Design review of the part built by this model. Coordinates are the model's own, in mm. A direction names the side the tool comes from. Coordinates: 2 decimals unless noted, no trailing zeros. Order: outer loops, then holes, each group sorted by start corner. A loop starts at its lowest first (then second) coordinate and runs counter-clockwise, first axis right, second up. Notation, with made-up numbers: M 31,-4.5 L 82,-4.5 A35 ccw 82,33.5 Z; hole C 25,16 d3. An arc over 180 degrees is marked long. Answer as a JSON object with one key per item and string values.
Autodesk Inventor part; units mm, degrees
ref_plane "Midplane" through (-32.0857, 98.175, 0) normal (0, -1, 0) x (1, 0, 0)
ref_plane "Work Plane3" through (-26.5857, 212.35, 16) normal (1, 0, 0) x (0, 0, -1)
ref_plane "YZ Plane" through (0, 0, 0) normal (1, 0, 0) x (0, 1, 0)
sketch "Sketch2" plane through (0, 0, 0) normal (0, 0, 1) x (1, 0, 0)
  line L0 (-32.0857, 0) -> (0, 0)
  line L1 (0, 0) -> (0, 19.635)
  line L2 (0, 19.635) -> (-32.0857, 19.635)
  spline S0 degree 3 poles (-32.0857, 19.635) (-32.0786, 19.6019) (-32.0585, 19.4984) (-32.0378, 19.3226) (-32.0222, 19.1083) (-32.0293, 18.8935) (-32.0484, 18.6795) (-32.102, 18.3981) (-32.1765, 18.0482) (-32.2416, 17.6965) (-32.2997, 17.416) (-32.364, 17.211) (-32.4396, 17.0099) (-32.536, 16.8179) (-32.6409, 16.6304) (-32.7641, 16.4543) (-32.8983, 16.2866) (-33.043, 16.1278) (-33.201, 15.9822) (-33.3669, 15.8459) (-33.5414, 15.7205) (-33.7857, 15.5713) (-34.1055, 15.4094) (-34.509, 15.2608) (-34.9249, 15.1525) (-35.3479, 15.078) (-35.7753, 15.0341) (-36.2047, 15.0215) (-36.6341, 15.0313) (-37.0623, 15.0646) (-37.3462, 15.1014) (-37.4881, 15.1198) knots -0.847201 -0.847201 -0.847201 -0.847201 -0.83705 -0.815587 -0.794126 -0.772659 -0.751201 -0.729734 -0.686802 -0.64387 -0.622403 -0.600945 -0.579478 -0.558017 -0.536554 -0.515088 -0.49363 -0.472163 -0.450698 -0.429238 -0.407769 -0.386302 -0.343394 -0.300476 -0.257562 -0.214646 -0.17172 -0.12879 -0.085861 -0.04293 0 0 0 0
  spline S1 degree 3 poles (-37.4881, 15.1198) (-37.594, 15.1249) (-37.8057, 15.1352) (-38.2295, 15.119) (-38.7575, 15.0717) (-39.3865, 14.9771) (-40.0103, 14.8535) (-40.6285, 14.7043) (-41.2408, 14.5326) (-41.847, 14.3405) (-42.4469, 14.1297) (-43.0405, 13.9015) (-43.6276, 13.6572) (-44.2081, 13.3977) (-44.782, 13.1239) (-45.3493, 12.8367) (-45.9097, 12.5363) (-46.4639, 12.2246) (-46.8275, 12.0066) (-47.0092, 11.8976) knots -1.017256 -1.017256 -1.017256 -1.017256 -0.985476 -0.953687 -0.890117 -0.826542 -0.762964 -0.699386 -0.635807 -0.572227 -0.508647 -0.445066 -0.381486 -0.317905 -0.254324 -0.190743 -0.127162 -0.063581 0 0 0 0
  arc A0 (-47.0092, 11.8976) -> (-47.0092, 7.7374) centre (9.2023, 9.8175) ccw
  spline S2 degree 3 poles (-47.0092, 7.7374) (-46.8275, 7.6284) (-46.4639, 7.4104) (-45.9097, 7.0987) (-45.3493, 6.7983) (-44.782, 6.5111) (-44.2081, 6.2373) (-43.6276, 5.9778) (-43.0405, 5.7335) (-42.4469, 5.5053) (-41.847, 5.2945) (-41.2408, 5.1024) (-40.6285, 4.9307) (-40.0103, 4.7815) (-39.3865, 4.6579) (-38.7575, 4.5633) (-38.2295, 4.516) (-37.8057, 4.4998) (-37.594, 4.5101) (-37.4881, 4.5152) knots -1.017256 -1.017256 -1.017256 -1.017256 -0.953675 -0.890094 -0.826513 -0.762932 -0.699351 -0.63577 -0.572189 -0.508609 -0.445029 -0.381449 -0.31787 -0.254291 -0.190714 -0.127139 -0.063568 -0.03178 0 0 0 0
  spline S3 degree 3 poles (-37.4881, 4.5152) (-37.3462, 4.5336) (-37.0623, 4.5704) (-36.6341, 4.6037) (-36.2047, 4.6135) (-35.7753, 4.6009) (-35.3479, 4.557) (-34.9249, 4.4825) (-34.509, 4.3742) (-34.1055, 4.2256) (-33.7857, 4.0637) (-33.5414, 3.9145) (-33.3669, 3.7891) (-33.201, 3.6528) (-33.043, 3.5072) (-32.8983, 3.3484) (-32.7641, 3.1807) (-32.6409, 3.0046) (-32.536, 2.8171) (-32.4396, 2.6251) (-32.364, 2.424) (-32.2997, 2.219) (-32.2416, 1.9385) (-32.1765, 1.5868) (-32.102, 1.2369) (-32.0484, 0.9555) (-32.0293, 0.7415) (-32.0222, 0.5267) (-32.0378, 0.3124) (-32.0585, 0.1366) (-32.0786, 0.0331) (-32.0857, 0) knots -1.373604 -1.373604 -1.373604 -1.373604 -1.330674 -1.287743 -1.244814 -1.201884 -1.158958 -1.116042 -1.073128 -1.03021 -0.987302 -0.965835 -0.944366 -0.922906 -0.901441 -0.879974 -0.858516 -0.83705 -0.815587 -0.794126 -0.772659 -0.751201 -0.729734 -0.686802 -0.64387 -0.622403 -0.600945 -0.579478 -0.558017 -0.536554 -0.526403 -0.526403 -0.526403 -0.526403
extrude "Extrusion1" add sketch "Sketch2" along normal blind 16
pattern_linear "Rectangular Pattern1" count 10 spacing 19.635 along (0, 1, 0) of "Extrusion1"
sketch "Sketch5" plane through (-32.0857, 0, 0) normal (0, -1, 0) x (1, 0, 0)
  line L0 (32.0857, 0) -> (32.0857, 16)
  line L1 (0, 16) -> (32.0857, 16)
  line L2 (0, 0) -> (32.0857, 0)
  line L3 (0, 0) -> (0, 16)
  line L4 (0, 16) -> (8, 16)
  line L5 (8, 16) -> (8, 0) construction
  line L6 (8, 0) -> (0, 0)
  line L7 (0, 0) -> (0, 16)
  line L8 (8, 16) -> (10.5, 16)
  line L9 (10.5, 16) -> (10.5, 10.5)
  line L10 (10.5, 10.5) -> (8, 10.5)
  line L11 (8, 10.5) -> (8, 16) construction
  line L12 (8, 2.5) -> (10.5, 2.5)
  line L13 (10.5, 2.5) -> (10.5, 0)
  line L14 (10.5, 0) -> (8, 0)
  line L15 (8, 0) -> (8, 2.5) construction
  line L16 (8, 9.5) -> (37, 9.5) construction
  line L17 (37, 9.5) -> (37, 3.5) construction
  line L18 (37, 3.5) -> (8, 3.5) construction
  line L19 (8, 3.5) -> (8, 9.5) construction
  line L20 (8, 10.5) -> (8, 2.5)
  line L21 (34.5, 15.5) -> (10.5, 15.5) construction
  line L22 (10.5, 15.5) -> (10.5, 0.5) construction
  line L23 (10.5, 0.5) -> (34.5, 0.5) construction
  line L24 (34.5, 0.5) -> (34.5, 15.5) construction
  line L25 (41.5759, 16) -> (41.5759, 15.5) construction
  line L26 (41.5759, 0.5) -> (41.5759, 0) construction
  line L27 (25.6, 16.05) -> (19.4, 16.05) construction
  line L28 (19.4, -0.05) -> (25.6, -0.05) construction
  line L29 (25.6, -0.05) -> (25.6, 0.5) construction
  line L30 (25.6, 15.5) -> (25.6, 16.05) construction
  line L31 (19.4, 16.05) -> (19.4, 15.5) construction
  line L32 (19.4, 0.5) -> (19.4, -0.05) construction
  line L33 (25.6, 0.5) -> (25.6, 15.5) construction
  line L34 (19.4, 15.5) -> (19.4, 0.5) construction
  point P0 (9.25, 10.5)
  point P1 (9.25, 2.5)
  point P2 (8, 6.5)
  point P3 (8, 6.5)
  point P4 (22.5, 15.5)
  point P5 (22.5, 9.5)
  point P6 (22.5, -0.05)
  dimension "d15" = 8
  dimension "d16" = 8
  dimension "d18" = 6
  dimension "d19" = 29
  dimension "d20" = 24
  dimension "d21" = 6
  dimension "d22" = 3
  dimension "d23" = 2.5
  dimension "d24" = 2.5
  dimension "d30" = 5.5
  dimension "d31" = 2.5
  dimension "d64" = 6.2
  dimension "d65" = 16.1
extrude "Extrusion3" cut sketch "Sketch5" against normal through all contours L2 L13 L12 L20 L10 L9 L1 L0
sketch "Measurements" plane through (0, 0, 0) normal (0, 0, -1) x (-1, 0, 0)
  line L0 (41.7977, 19.635) -> (70.5831, 19.635) construction
  line L1 (141.7977, 176.7146) -> (141.7977, 118.484) construction
  line L2 (21.5857, 196.35) -> (21.5857, 0)
  line L3 (32.0857, 0) -> (21.5857, 0)
  circle A0 centre (91.7977, 19.635) radius 50 construction
  line L4 (41.7977, -40.4843) -> (41.7977, 79.7543) construction
  line L5 (41.7977, 19.635) -> (141.7977, 19.635) construction
  line L6 (141.7977, 19.635) -> (141.7977, 176.7146) construction
  arc A1 (41.7977, 19.635) -> (141.7977, 176.7146) centre (-31.5724, 176.7146) ccw construction
  circle A2 centre (91.7977, 176.7146) radius 50 construction
  line L7 (-14.9143, 139.9646) -> (32.0857, 139.9646) construction
  line L8 (32.0857, 139.9646) -> (32.0857, 213.4646) construction
  line L9 (32.0857, 213.4646) -> (-14.9143, 213.4646) construction
  line L10 (-14.9143, 213.4646) -> (-14.9143, 139.9646) construction
  circle A3 centre (91.7977, 176.7146) radius 5 construction
  line L11 (32.0857, 139.9646) -> (96.4406, 164.572) construction
  arc A4 (96.4406, 164.572) -> (96.4406, 188.8572) centre (91.7977, 176.7146) ccw construction
  line L12 (96.4406, 188.8572) -> (32.0857, 213.4646) construction
  line L13 (-14.9143, -17.115) -> (32.0857, -17.115) construction
  line L14 (32.0857, -17.115) -> (32.0857, 56.385) construction
  line L15 (32.0857, 56.385) -> (-14.9143, 56.385) construction
  line L16 (-14.9143, 56.385) -> (-14.9143, -17.115) construction
  circle A5 centre (91.7977, 19.635) radius 5 construction
  line L17 (32.0857, -17.115) -> (96.4406, 7.4924) construction
  arc A6 (96.4406, 7.4924) -> (96.4406, 31.7776) centre (91.7977, 19.635) ccw construction
  line L18 (96.4406, 31.7776) -> (32.0857, 56.385) construction
  line L19 (96.7977, 176.7146) -> (96.7977, 157.197) construction
  line L20 (96.7977, 19.635) -> (96.7977, 0.1424) construction
  circle A7 centre (9.5857, 201.4646) radius 14.5 construction
  line L21 (-14.9143, 176.7146) -> (-21.6792, 176.7146)
  circle A8 centre (9.5857, 151.9646) radius 14.5 construction
  point P0 (0, 0)
  point P1 (32.0857, 176.7146)
  point P2 (104.7977, 176.7146)
  point P3 (104.7977, 19.635)
  point P4 (32.0857, 19.635)
  dimension "d43" = 10
  dimension "d32" = 100
  dimension "d33" = 157.0796
  dimension "d34" = 59.712
  dimension "d36" = 73.5
  dimension "d37" = 47
  dimension "d38" = 73.5
  dimension "d39" = 47
  dimension "d41" = 8
  dimension "d44" = 17.115
  dimension "d66" = 29
  dimension "d67" = 12
  dimension "d68" = 24.5
ref_plane "Midplane" through (-32.0857, 98.175, 0) normal (0, -1, 0) x (1, 0, 0)
sketch "Sketch10" plane through (-32.0857, 196.35, 16) normal (0, 1, 0) x (1, 0, 0)
  line L0 (0, 16) -> (0, 0)
  line L1 (10.5, 16) -> (0, 16)
  line L2 (0, 16) -> (10.5, 16)
  line L3 (10.5, 13.5) -> (10.5, 16)
  line L4 (10.5, 13.5) -> (8, 13.5)
  line L5 (8, 13.5) -> (10.5, 13.5)
  line L6 (8, 13.5) -> (8, 5.5)
  line L7 (8, 5.5) -> (8, 13.5)
  line L8 (8, 5.5) -> (10.5, 5.5)
  line L9 (10.5, 5.5) -> (8, 5.5)
  line L10 (10.5, 5.5) -> (10.5, 0)
  line L11 (10.5, 0) -> (0, 0)
  line L12 (0, 0) -> (0, 16)
  point P0 (32.0857, 16)
extrude "Extra" add sketch "Sketch10" along normal blind 18
sketch "Sketch11" plane through (-32.0857, 214.35, 16) normal (0, 1, 0) x (1, 0, 0)
  line L0 (0, 16) -> (15.5, 16)
  line L1 (15.5, 16) -> (15.5, 0)
  line L2 (15.5, 0) -> (0, 0)
  line L3 (0, 0) -> (0, 16)
  line L4 (0, 0) -> (10.5, 0)
  line L5 (10.5, 16) -> (0, 16)
  line L6 (10.5, 0) -> (10.5, 5.5)
  line L7 (0, 16) -> (0, 0)
  point P0 (32.0857, 16)
  dimension "d63" = 5
extrude "Bracket" add sketch "Sketch11" along normal blind 16
sketch "Sketch13" plane through (-16.5857, 214.35, 16) normal (1, 0, 0) x (0, 0, -1)
  circle A0 centre (8, 8) radius 5.865
  line L0 (16, 0) -> (16, 16)
  line L1 (0, 16) -> (16, 16)
  point P0 (16, -214.35)
  point P1 (16, 8)
  point P2 (8, 16)
  dimension "d69" = 11.73
hole "Hole1" at (-16.5857, 222.35, 8) direction (-1, 0, 0) diameter 6 end through all countersink diameter 13.44 countersink angle 90
fillet "Fillet2" radius 2 3 edges at (-21.5857, 214.35, 1.25) (-24.0857, 214.35, 6.5) (-21.5857, 214.35, 13.25)
mirror "Mirror3" about plane through (-32.0857, 98.175, 0) normal (0, -1, 0) of "Fillet2", "Hole1", "Bracket", "Extra"
ref_plane "Work Plane3" through (-26.5857, 212.35, 16) normal (1, 0, 0) x (0, 0, -1)
sketch "Sketch14" plane through (-26.5857, 212.35, 16) normal (1, 0, 0) x (0, 0, -1)
  line L0 (26.8583, 24.8606) -> (-9.9213, 24.8606)
  line L1 (-9.9213, 24.8606) -> (-9.9213, -261.2458)
  line L2 (-9.9213, -261.2458) -> (26.8583, -261.2458)
  line L3 (26.8583, -261.2458) -> (26.8583, 24.8606)
  point P0 (16, -212.35)
extrude "Extrusion7" cut sketch "Sketch14" against normal through all
sketch "Sketch15" plane through (-24.0857, 212.35, 10.5) normal (1, 0, 0) x (0, 0, -1)
  circle A0 centre (4, -223.35) radius 3
  line L0 (-47.7239, -114.175) -> (-79.2168, -114.175)
  line L1 (-32.3539, 18) -> (-32.3539, -246.35) construction
  circle A1 centre (4, -5) radius 3
  line L2 (8, 2) -> (0, 2)
  line L3 (8, -228.35) -> (0, -228.35)
  line L4 (-5.5, -246.35) -> (10.5, -246.35)
  point P0 (0, 18)
  point P1 (-32.3539, -114.175)
  point P2 (4, 2)
  point P3 (-5.5, 18)
  dimension "d82" = 6
  dimension "d83" = 5
  dimension "d86" = 23
  dimension "d87" = 9.5
extrude "Extrusion8" cut sketch "Sketch15" against normal through all
properties part number "rack6mm-v2-top"
1) Add section B-B (y = 12.5). State the section outline as (x, z) points, and give its area (3 significant figures).
Taken from the geometry:
{"outline": "M -26.59,0 L -21.59,0 L -21.59,2.5 L -24.09,2.5 L -24.09,10.5 L -21.59,10.5 L -21.59,16 L -26.59,16 Z", "area": "60.0 mm2"}
2) Mouldability with a two-part tool opening along Y and no side actions: class faces 3 (the flat face through (-24, 100, 0)), 4 (the flat face through (-22, 230.35, 8)), 5 (the flat face through (-21.586, 100, 13)) as released by +Y, released by -Y, zero draft, split by the parting line, or undercut.
Taken from the geometry:
{"face 3": "zero draft", "face 4": "released by +Y", "face 5": "undercut"}
3) Add section A-A (y = 222.35). State the section outline as (x, z) points, and give its area (3 significant figures).
Taken from the geometry:
{"outline": "M -26.59,0 L -16.59,0 L -16.59,1.28 L -20.31,5 L -26.59,5 Z; M -26.59,11 L -20.31,11 L -16.59,14.72 L -16.59,16 L -26.59,16 Z", "area": "86.2 mm2"}
4) To check wall thickness, follow L1, parallel to Y at x = -21.75, z = 8; L2, parallel to Z at x = -24, y = 202; L3, parallel to Z at x = -24, y = -26. State the ranges of each line that lie inside material, in increasing order.
Taken from the geometry:
{"L1": "y = -34 to -29, -23 to -18, 214.35 to 219.35, 225.35 to 230.35", "L2": "z = 0 to 2.5, 10.5 to 16", "L3": "z = 0 to 5, 11 to 16"}
5) Insertion check: pin 1 Ø9 at (y, z) = (98.5, 5) entering from +X; pin 2 Ø1.5 at (y, z) = (155.5, 6) entering from +X. Each pin has a flat end and moves straight along its axis. Give the tip position at first contact, or say it passes through.
Taken from the geometry:
{"pin 1": "stops at x = -21.59", "pin 2": "stops at x = -24.09"}
6) Tool access review of faces 1 (the flat face through (-19, -18, 8)), 2 (the cylindrical face through (-23.49, -24.85, 5.23)): name each direction out of +Z, -Z, +X, -X, +Y, -Y from which nothing blocks a thin tool from reaching the whole face with its end or side.
Taken from the geometry:
{"face 1": "+X", "face 2": "+X, -X"}
